Geometry: final body of the model. Coordinates: model frame, mm. Face numbers are marked on the shaded views. A direction names the side the tool comes from. Give positions to 0.01 mm unless a question says otherwise; leave off trailing zeros. Loops run counter-clockwise (first coordinate to the right, second up) from the corner with the lowest first, then second, coordinate; pieces in that order, holes last.
1. First-contact query: P1, Ø4, axis at x = 2.5, y = -32.5, coming from the -Z side; P2, Ø3.5, axis at x = 32.5, y = -17.5, coming from the +Z side; P3, Ø10, axis at y = 14, z = 18, coming from the +X side; P4, Ø5.5, axis at x = -19.98, y = 34.6, coming from the +Z side. Flat tips, straight axial feed; report the tip coordinate or a pass-through.
2. Section D-D, the plane z = 10.75. Output: boundary loops of the cut face in (x, y).
3. Section C-C, the plane x = 35.5. Output: boundary loops of the cut face in (y, z), then the cut area to 3 significant figures.
4. Access query for the marked faces 1, 2 and 3. Directions: +Z, -Z, +X, -X, +Y, -Y. A direction counts if a zero-diameter tool reaches every point of the face in a straight line with its end or side. Return the directions, or none.
5. Draft query along Y for the marked faces 4, 5 and 6. Return one class per face: +Y half, -Y half, draft (parallel to the pull), parting line (faces both ways), or undercut.
6. Material intervals for line 1 along X through (y, z) = (35.5, 14.75); line 2 along Y through (x, z) = (0, 13.25); line 3 along X through (y, z) = (-21.5, 19.25), sorted ascending.
7. Section A-A, the plane y = 0. Output: boundary loops of the cut face in (x, z) (3 decimals), then the cut area to 3 significant figures.
from build123d import *

# Parameters (mm, degrees)
F3_D           = 6.6
F3_DEPTH       = 35
F3_CBORE_D     = 11.25
F3_CBORE_DEPTH = 6
F3_TIP         = 1.9828400428
F5_D           = 17.5
F5_DEPTH       = 39.5
F5_TIP         = 5.2575304165


with BuildPart() as f1:
    # F0 (on Front) → F1 (revolve)
    with BuildSketch(Plane.XZ):
        Polygon((-29.9, 14), (-29.9, 0), (0, 0), (0, 25), (-49.95, 25), (-49.95, 14), align=None)
    revolve(axis=Axis((0, 0, 12.5), (0, 0, -1)))

    # F3
    with Locations(Plane.XY.offset(25)):
        with Locations((19.975, -34.5977148812), (39.95, 0), (34.5977148812, 19.975), (34.5977148812, -19.975), (19.975, 34.5977148812), (0, 39.95), (-19.975, 34.5977148812), (-34.5977148812, 19.975), (-39.95, 0), (-34.5977148812, -19.975), (-19.975, -34.5977148812), (0, -39.95)):
            CounterBoreHole(F3_D / 2, F3_CBORE_D / 2, F3_CBORE_DEPTH, depth=F3_DEPTH)
            with Locations((0, 0, -(F3_DEPTH + F3_TIP / 2))):  # 118° drill point
                Cone(0, F3_D / 2, F3_TIP, mode=Mode.SUBTRACT)

    # F5
    with Locations(Plane.XY.offset(25)):
        with Locations((0, 0)):
            Hole(F5_D / 2, depth=F5_DEPTH)
            with Locations((0, 0, -(F5_DEPTH + F5_TIP / 2))):  # 118° drill point
                Cone(0, F5_D / 2, F5_TIP, mode=Mode.SUBTRACT)


solid = f1.part
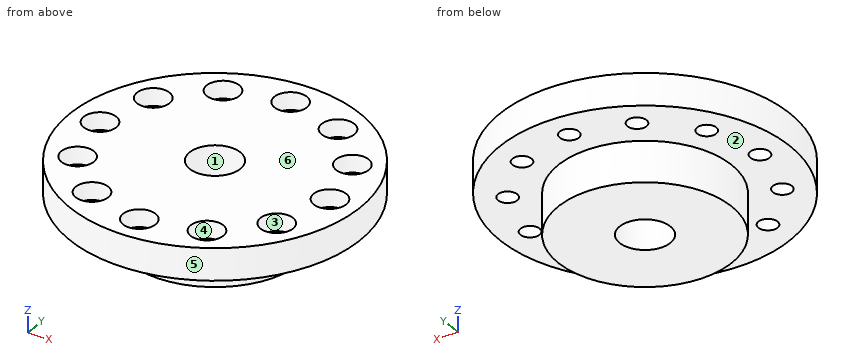
Answers below:
1. P1: stops at z = 14
1. P2: stops at z = 19
1. P3: stops at x = 49.13
1. P4: passes through
2. outline: circle Ø59.8 at (0, 0); hole circle Ø17.5 at (0, 0)
3. outline: (-35.14, 14) - (-23.15, 14) - (-23.15, 19) - (-25.53, 19) - (-25.53, 25) - (-35.14, 25) - close; (-16.8, 14) - (16.8, 14) - (16.8, 19) - (14.42, 19) - (14.42, 25) - (3.44, 25) - (3.44, 19) - (-3.44, 19) - (-3.44, 25) - (-14.42, 25) - (-14.42, 19) - (-16.8, 19) - close; (23.15, 14) - (35.14, 14) - (35.14, 25) - (25.53, 25) - (25.53, 19) - (23.15, 19) - close
3. area: 535 mm2
4. face 1: +Z, -Z
4. face 2: -Z
4. face 3: +Z
5. face 4: undercut
5. face 5: parting line
5. face 6: draft
6. line 1: x = -35.14 to -23.15, -16.8 to 16.8, 23.15 to 35.14
6. line 2: y = -29.9 to -8.75, 8.75 to 29.9
6. line 3: x = -45.09 to -40.01, -29.18 to 29.18, 40.01 to 45.09
7. outline: (-49.95, 14) - (-43.25, 14) - (-43.25, 19) - (-45.575, 19) - (-45.575, 25) - (-49.95, 25) - close; (-36.65, 14) - (-29.9, 14) - (-29.9, 0) - (-8.75, 0) - (-8.75, 25) - (-34.325, 25) - (-34.325, 19) - (-36.65, 19) - close; (8.75, 0) - (29.9, 0) - (29.9, 14) - (36.65, 14) - (36.65, 19) - (34.325, 19) - (34.325, 25) - (8.75, 25) - close; (43.25, 14) - (49.95, 14) - (49.95, 25) - (45.575, 25) - (45.575, 19) - (43.25, 19) - close
7. area: 1,300 mm2
